Check sheet for the drawn part. Datum: minimum x, y, z corner. Units: mm. A direction names the side the tool comes from. Give positions to 0.01 mm unless a question says otherwise; leave off trailing zeros. Write each loop counter-clockwise with the first axis right and the second up, starting at its lowest first coordinate (ties: lowest second). Pieces come first, ordered by that corner, then holes.
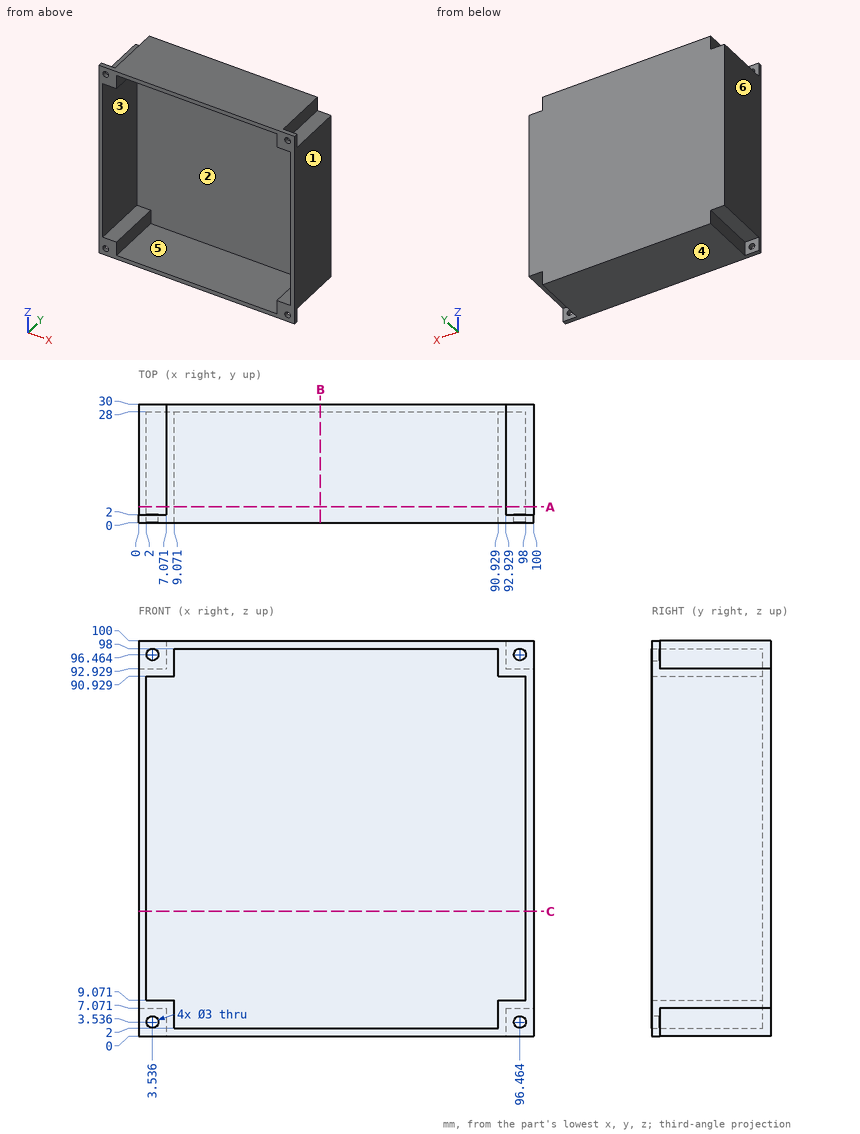
1) Sectioned sample at B-B on x = 46. Record the boundary of the cut face in (y, z).
2) Sectioned sample at C-C on z = 31.5. Record the boundary of the cut face in (x, y), then the cut area to 3 significant figures.
3) Scan lines: L1, parallel to Z at x = 17, y = 16.25; L2, parallel to Z at x = 4.5, y = 7.75. Record each from-to range of solid material in increasing order.
4) Draft check along Z on the marked faces 1, 2, 3 and 4. Enter one of: +Z half, -Z half, draft (parallel to the pull), parting line (faces both ways), or undercut.
5) Access from +Z, -Z, +X, -X, +Y, -Y to the whole of each face (thin tool, end or side, straight path). Record for the marked faces 5 and 6.
6) Sectioned sample at A-A on y = 4. Record the boundary of the cut face in (x, z).
7) Gauge pin test, flat ends, axial feed: pin 1 (2 mm diameter, centred on x = 4, z = 95, fed in from +Y); pin 2 (3.5 mm diameter, centred on y = 7, z = 95, fed in from +X); pin 3 (3.5 mm diameter, centred on y = 15, z = 97, fed in from -X). Record the tip position at first contact, or that the pin passes through.
Answers below:
1. outline: (0, 0) - (30, 0) - (30, 100) - (0, 100) - (0, 98) - (28, 98) - (28, 2) - (0, 2) - close
2. outline: (0, 0) - (2, 0) - (2, 28) - (98, 28) - (98, 0) - (100, 0) - (100, 30) - (0, 30) - close
2. area: 312 mm2
3. L1: z = 0 to 2, 98 to 100
3. L2: z = 7.07 to 9.07, 90.93 to 92.93
4. face 1: draft
4. face 2: undercut
4. face 3: undercut
4. face 4: -Z half
5. face 5: -Y
5. face 6: +Z, -Z, -X, +Y, -Y
6. outline: (0, 7.07) - (7.07, 7.07) - (7.07, 0) - (92.93, 0) - (92.93, 7.07) - (100, 7.07) - (100, 92.93) - (92.93, 92.93) - (92.93, 100) - (7.07, 100) - (7.07, 92.93) - (0, 92.93) - close; hole (2, 9.07) - (9.07, 9.07) - (9.07, 2) - (90.93, 2) - (90.93, 9.07) - (98, 9.07) - (98, 90.93) - (90.93, 90.93) - (90.93, 98) - (9.07, 98) - (9.07, 90.93) - (2, 90.93) - close
7. pin 1: stops at y = 2
7. pin 2: stops at x = 92.93
7. pin 3: stops at x = 7.07
